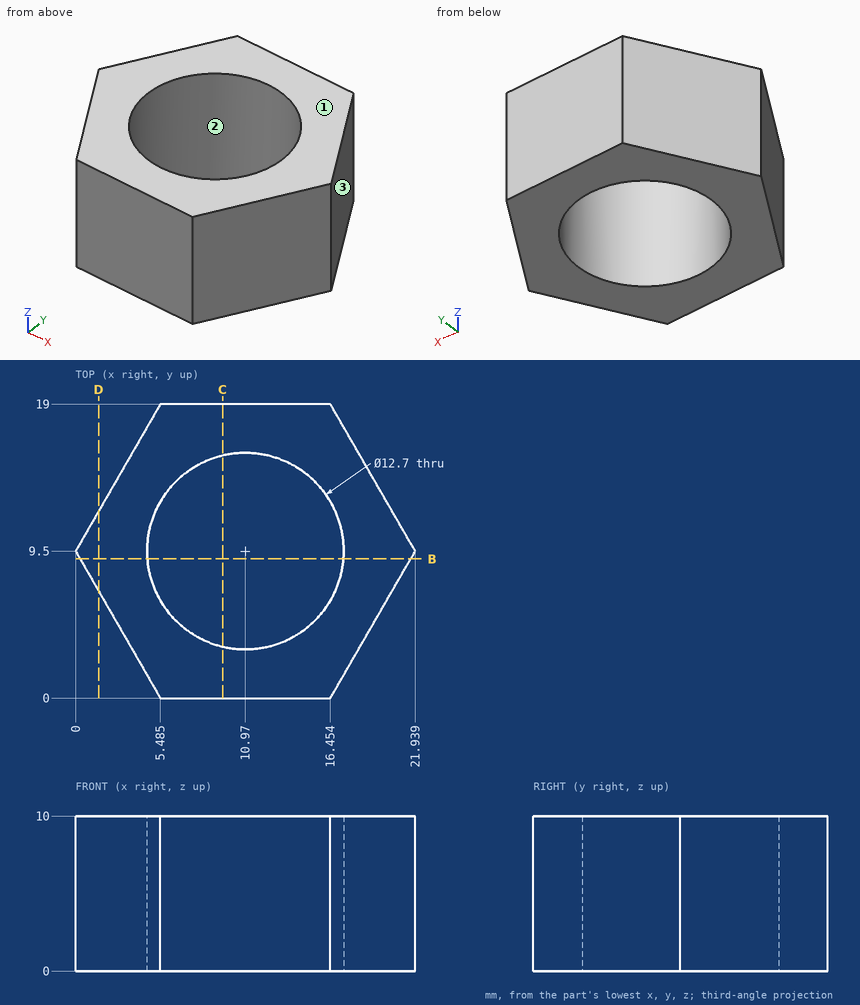
Geometry check sheet. Reference: drawing and pictorial views, mm from the part's lowest x, y, z. Give positions to 0.01 mm unless a question says otherwise; leave off trailing zeros. Write each loop counter-clockwise with the first axis right and the second up, starting at its lowest first coordinate (ties: lowest second). Pieces come first, ordered by that corner, then holes. Notation, with made-up numbers: (75, 70) -> (95, 70) arc R21 cw to (95, 84) -> close; hole circle Ø4 at (5, 14.5). An arc over 180 degrees is marked (long way). One line per item, written item: value. Start each with the question number.
Item 1: Material ranges on probe 1 along X at (y, z) = (12.75, 1) (1 decimal); probe 2 along Y at (x, z) = (5.5, 4.25) (1 decimal); probe 3 along X at (y, z) = (1.5, 9), recorded low to high. Write a range as from..to.
Item 2: Draft check along X on the marked faces 1, 2 and 3. Enter one of: +X half, -X half, draft (parallel to the pull), parting line (faces both ways), or undercut.
Item 3: Gauge pin test, flat ends, axial feed: pin 1 (1 mm diameter, centred on x = 17, y = 2.5, fed in from -Z); pin 2 (6 mm diameter, centred on x = 19.5, z = 3.5, fed in from +Y). Record the tip position at first contact, or that the pin passes through.
Item 4: Section check B-B on y = 9. Record the cut outline in (x, z).
Item 5: Section check D-D on x = 1.5. Record the cut outline in (y, z).
Item 6: Section check C-C on x = 9.5. Record the cut outline in (y, z).
Results list:
1. probe 1: 1.9..5.5, 16.4..20.1
1. probe 2: 0..6.3, 12.7..19
1. probe 3: 4.62..17.32
2. face 1: draft
2. face 2: undercut
2. face 3: +X half
3. pin 1: z = 0
3. pin 2: y = 18.92
4. outline: (0.29, 0) -> (4.64, 0) -> (4.64, 10) -> (0.29, 10) -> close; (17.3, 0) -> (21.65, 0) -> (21.65, 10) -> (17.3, 10) -> close
5. outline: (6.9, 0) -> (12.1, 0) -> (12.1, 10) -> (6.9, 10) -> close
6. outline: (0, 0) -> (3.32, 0) -> (3.32, 10) -> (0, 10) -> close; (15.68, 0) -> (19, 0) -> (19, 10) -> (15.68, 10) -> close
